```python
from build123d import *

# Parameters (mm, degrees)
SHELL4_T            = -2.5
SKETCH5_W           = 5.8
SKETCH5_H           = 4
BOSS_EXTRUDE1_DEPTH = 10.9
CUT_EXTRUDE3_DEPTH  = 4
SKETCH7_W           = 12
SKETCH7_H           = 6
CUT_EXTRUDE4_DEPTH  = 0.3


with BuildPart() as part:
    # Sketch1 → Loft2 section 0
    with BuildSketch(Plane.XY):
        with BuildLine():
            Line((-9.05, 9.05), (9.05, 9.05))
            Line((9.05, 9.05), (9.05, -9.05))
            Line((9.05, -9.05), (-9.05, -9.05))
            Line((-9.05, -9.05), (-9.05, 9.05))
        make_face()
    # Sketch2 → Loft2 section 1
    with BuildSketch(Plane.XY.offset(9.4)):
        with BuildLine():
            Line((-6.185, 6.185), (6.185, 6.185))
            Line((6.185, 6.185), (6.185, -6.185))
            Line((6.185, -6.185), (-6.185, -6.185))
            Line((-6.185, -6.185), (-6.185, 6.185))
        make_face()
    loft()

    # Shell4
    shell4_openings = [part.faces().sort_by_distance(p)[0] for p in [
        (0, 0, 0),
    ]]
    offset(amount=SHELL4_T, openings=shell4_openings, kind=Kind.INTERSECTION)

    # Sketch5 → Boss-Extrude1 (add)
    with BuildSketch(Plane.XY.offset(-4)):
        Rectangle(SKETCH5_W, SKETCH5_H)
    extrude(amount=BOSS_EXTRUDE1_DEPTH)

    # Sketch6 → Cut-Extrude3 (cut)
    with BuildSketch(Plane(origin=(0, 0, -4), x_dir=(-1, 0, 0), z_dir=(0, 0, -1))):
        Polygon((0.73, 2.15), (-0.73, 2.15), (-0.73, 0.73), (-2.15, 0.73), (-2.15, -0.73), (-0.73, -0.73), (-0.73, -2.15), (0.73, -2.15), (0.73, -0.73), (2.15, -0.73), (2.15, 0.73), (0.73, 0.73), align=None)
    extrude(amount=-CUT_EXTRUDE3_DEPTH, mode=Mode.SUBTRACT)

    # Sketch7 → Cut-Extrude4 (cut)
    with BuildSketch(Plane(origin=(0, -8.280756947, 2.523869006), x_dir=(1, 0, 0), z_dir=(0, -0.9565567247121477, 0.2915462783298196))):
        with Locations((0, 2.765838851)):
            Rectangle(SKETCH7_W, SKETCH7_H)
    extrude(amount=-CUT_EXTRUDE4_DEPTH, mode=Mode.SUBTRACT)


solid = part.part
```
Here's how the part is built. I have some questions about the finished solid (model axes, mm). A direction names the side the tool comes from. Coordinates: 2 decimals unless noted, no trailing zeros. Order: outer loops, then holes, each group sorted by start corner. A loop starts at its lowest first (then second) coordinate and runs counter-clockwise, first axis right, second up. Notation, with made-up numbers: M -28,30.25 L -5,30.25 A28 ccw -5,66.25 Z; hole C 57,21 d3. An arc over 180 degrees is marked long. Answer as a JSON object with one key per item and string values. Group by question number.
(1) I need wall thicknesses on probe 1 along Y at (x, z) = (2, -1.5); probe 2 along X at (y, z) = (1, 3); probe 3 along X at (y, z) = (1, 1). Which ranges of each line are inside material? Lowest first, please.
(2) If we mould it in two halves opening along X, with no side actions, what happens to faces 1 (the face through (-2.15, 0, -2)), 2 (the face through (-7, 0, 0))? For each: released by +X, released by -X, zero draft, split by the parting line, or undercut.
(3) Suppose I cut it at B-B, the plane z = 3. State how many separate pieces and enclosed holes the cut face has, then the cut area to 3 significant figures.
(4) For pin 1 (1 mm diameter, centred on y = -7.5, z = 5.5, fed in from +X); pin 2 (1.7 mm diameter, centred on x = 0.5, z = 0.5, fed in from -Y); pin 3 (1.4 mm diameter, centred on y = -1.5, z = -3, fed in from +X); pin 4 (0.6 mm diameter, centred on y = 1.5, z = -2.5, fed in from -X), each with a flat end and sliding along its axis, tell me the tip position at first contact or that it passes through.
(5) Which directions (+Z, -Z, +X, -X, +Y, -Y) give clear straight access to the entire face, cutting with the end or side of a thin tool? Please do faces 3 (the face through (0.73, 1, -2)), 4 (the face through (-0.09, 5.37, 3.5)), 5 (the face through (-2.31, 0.03, -4)).
(6) Suppose I cut it at A-A, the plane z = -1.75. Please give me the cut outline in (x, y).
Values found:
{
 "1": {"probe 1": "y = -2 to -0.73, 0.73 to 2", "probe 2": "x = -8.14 to -5.52, -2.9 to 2.9, 5.52 to 8.14", "probe 3": "x = -8.75 to -6.13, -2.9 to 2.9, 6.13 to 8.75"},
 "2": {"face 1": "undercut", "face 2": "zero draft"},
 "3": {"separate pieces": "2", "enclosed holes": "1", "area": "162 mm^2"},
 "4": {"pin 1": "stops at x = 7.53", "pin 2": "stops at y = -9.05", "pin 3": "stops at x = 2.9", "pin 4": "stops at x = -2.9"},
 "5": {"face 3": "-Z, +Y, -Y", "face 4": "-Z", "face 5": "-Z, +X, -X, +Y, -Y"},
 "6": {"outline": "M -2.9,-2 L -0.73,-2 L -0.73,-0.73 L -2.15,-0.73 L -2.15,0.73 L -0.73,0.73 L -0.73,2 L -2.9,2 Z; M 0.73,-2 L 2.9,-2 L 2.9,2 L 0.73,2 L 0.73,0.73 L 2.15,0.73 L 2.15,-0.73 L 0.73,-0.73 Z"}
}
